```python
from build123d import *

# Parameters (mm, degrees)
SKETCH1_R           = 12.5
BOSS_EXTRUDE1_DEPTH = 50
BOSS_EXTRUDE2_DEPTH = 10
BOSS_EXTRUDE3_DEPTH = 14
SKETCH4_R           = 12.5
BOSS_EXTRUDE4_DEPTH = 50


with BuildPart() as part:
    # Sketch1 → Boss-Extrude1 (new, symmetric)
    with BuildSketch(Plane.XY):
        Circle(SKETCH1_R)
    extrude(amount=BOSS_EXTRUDE1_DEPTH, both=True)

    # Sketch2 → Boss-Extrude2 (add)
    with BuildSketch(Plane.XY.offset(50)):
        with BuildLine():
            Line((0, -135), (50, -135))
            ThreePointArc((50, -135), (57.725254986, -58.987850945), (42.132117825, 15.807740116))
            ThreePointArc((42.132117825, 15.807740116), (-11.798039133, 43.425871006), (-44.338945511, -7.684914504))
            ThreePointArc((-44.338945511, -7.684914504), (-45.875603416, -66.642123234), (-70, -120.459660044))
            Line((-70, -120.459660044), (-70, -135))
            Line((-70, -135), (0, -135))
        make_face()
    boss_extrude2 = extrude(amount=BOSS_EXTRUDE2_DEPTH)

    # Mirror1: Boss-Extrude2 across plane
    add(boss_extrude2.mirror(Plane.XY))

    # Sketch3 → Boss-Extrude3 (add)
    with BuildSketch(Plane(origin=(0, -135, 0), x_dir=(-1, 0, 0), z_dir=(0, -1, 0))):
        with BuildLine():
            Line((120, 7), (104.77406241, 7))
            ThreePointArc((104.77406241, 7), (101.238528504, 5.535533906), (99.77406241, 2))
            Line((99.77406241, 2), (99.77406241, -2))
            ThreePointArc((99.77406241, -2), (101.238528504, -5.535533906), (104.77406241, -7))
            Line((104.77406241, -7), (120, -7))
            ThreePointArc((120, -7), (123.535533906, -8.464466094), (125, -12))
            Line((125, -12), (125, -17))
            ThreePointArc((125, -17), (123.535533906, -20.535533906), (120, -22))
            Line((120, -22), (104.77406241, -22))
            ThreePointArc((104.77406241, -22), (101.238528504, -23.464466094), (99.77406241, -27))
            Line((99.77406241, -27), (99.77406241, -30))
            ThreePointArc((99.77406241, -30), (101.238528504, -33.535533906), (104.77406241, -35))
            Line((104.77406241, -35), (120, -35))
            ThreePointArc((120, -35), (123.535533906, -36.464466094), (125, -40))
            Line((125, -40), (125, -45))
            ThreePointArc((125, -45), (123.535533906, -48.535533906), (120, -50))
            Line((120, -50), (-50, -50))
            Line((-50, -50), (-50, 50))
            Line((-50, 50), (120, 50))
            ThreePointArc((120, 50), (123.535533906, 48.535533906), (125, 45))
            Line((125, 45), (125, 40))
            ThreePointArc((125, 40), (123.535533906, 36.464466094), (120, 35))
            Line((120, 35), (104.77406241, 35))
            ThreePointArc((104.77406241, 35), (101.238528504, 33.535533906), (99.77406241, 30))
            Line((99.77406241, 30), (99.77406241, 27))
            ThreePointArc((99.77406241, 27), (101.238528504, 23.464466094), (104.77406241, 22))
            Line((104.77406241, 22), (120, 22))
            ThreePointArc((120, 22), (123.535533906, 20.535533906), (125, 17))
            Line((125, 17), (125, 12))
            ThreePointArc((125, 12), (123.535533906, 8.464466094), (120, 7))
        make_face()
    extrude(amount=-BOSS_EXTRUDE3_DEPTH)

    # Sketch4 → Boss-Extrude4 (add)
    with BuildSketch(Plane(origin=(0, -135, 0), x_dir=(-1, 0, 0), z_dir=(0, -1, 0))):
        with Locations(Location((0, 0, 0), (0, 0, 270))):
            Circle(SKETCH4_R)
    extrude(amount=BOSS_EXTRUDE4_DEPTH)


solid = part.part
```
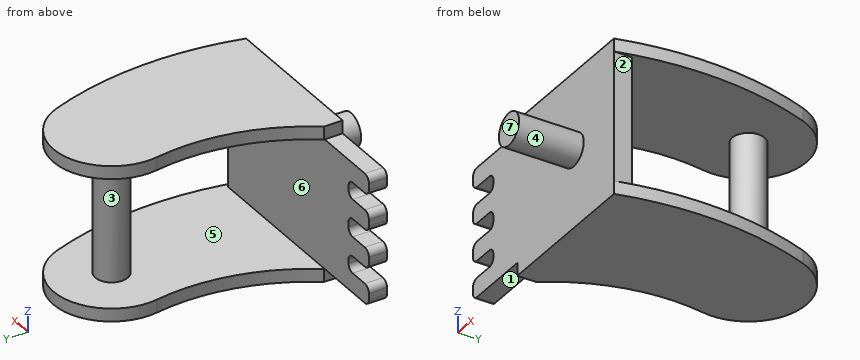
Check sheet for the modelled part. Datum: model origin and axes. Units: mm. Face numbers are marked on the shaded views. A direction names the side the tool comes from. Coordinates: 2 decimals unless noted, no trailing zeros. Loops run counter-clockwise (first coordinate to the right, second up) from the corner with the lowest first, then second, coordinate; pieces in that order, holes last. Notation, with made-up numbers: M -2.75,-40 L 55.25,-40 A16 cw 55.25,-16 Z; hole C 86.5,72.5 d6. An arc over 180 degrees is marked long. Answer as a JSON object with one key per item and string values.
1. Access from +Z, -Z, +X, -X, +Y, -Y to the whole of each face (thin tool, end or side, straight path). Record for the marked faces 1, 2 and 3.
Outcome:
{"face 1": "-Z, -X, +Y, -Y", "face 2": "+X, +Y, -Y", "face 3": "none"}
2. Scan lines: L1, parallel to Z at x = -48, y = -98; L2, parallel to Y at x = -31.5, z = -6; L3, parallel to Y at x = -6.5, z = 1.5. Record each from-to range of solid material in increasing order. Write a range as from..to.
Outcome:
{"L1": "-60..-50, 50..60", "L2": "-135..-121", "L3": "-185..-121, -10.68..10.68"}
3. Sectioned sample at A-A on x = 0. Record the cut outline in (y, z), and give its area (3 significant figures).
Outcome:
{"outline": "M -185,-12.5 L -135,-12.5 L -135,-60 L 45,-60 L 45,-50 L 12.5,-50 L 12.5,50 L 45,50 L 45,60 L -135,60 L -135,12.5 L -185,12.5 Z; hole M -121,-50 L -12.5,-50 L -12.5,50 L -121,50 Z", "area": "8,750 mm²"}
4. Sectioned sample at D-D on y = -166. Record the cut outline in (x, z), and give its area (3 significant figures).
Outcome:
{"outline": "C 0,0 d25", "area": "491 mm²"}
5. Sectioned sample at B-B on y = -114.5. Record the cut outline in (x, z), and give its area (3 significant figures).
Outcome:
{"outline": "M -65.97,-60 L 54.43,-60 L 54.43,-50 L -65.97,-50 Z; M -65.97,50 L 54.43,50 L 54.43,60 L -65.97,60 Z", "area": "2,410 mm²"}
6. Release check for a two-part mould opening along Z. For the marked faces 4, 5, 6 and 7 record: pulls with the +Z half, pulls with the -Z half, needs draft (parallel to the pull), parting line crosses it, or undercut.
Outcome:
{"face 4": "parting line crosses it", "face 5": "undercut", "face 6": "undercut", "face 7": "needs draft"}
7. Sectioned sample at C-C on x = -49. Record the cut outline in (y, z).
Outcome:
{"outline": "M -135,-60 L -78.22,-60 L -78.22,-50 L -121,-50 L -121,50 L -78.22,50 L -78.22,60 L -135,60 Z"}
8. Depth check by flat-ended pin: P1, Ø6, axis at x = -22, z = 24.5, coming from the +Y side; P2, Ø4, axis at x = -109.5, y = -129, coming from the +Z side; P3, Ø1, axis at y = -128, z = -23.5, coming from the +X side. Enter the tip coordinate at first touch or a pass-through.
Outcome:
{"P1": "y = -121", "P2": "z = 50", "P3": "x = 50"}
